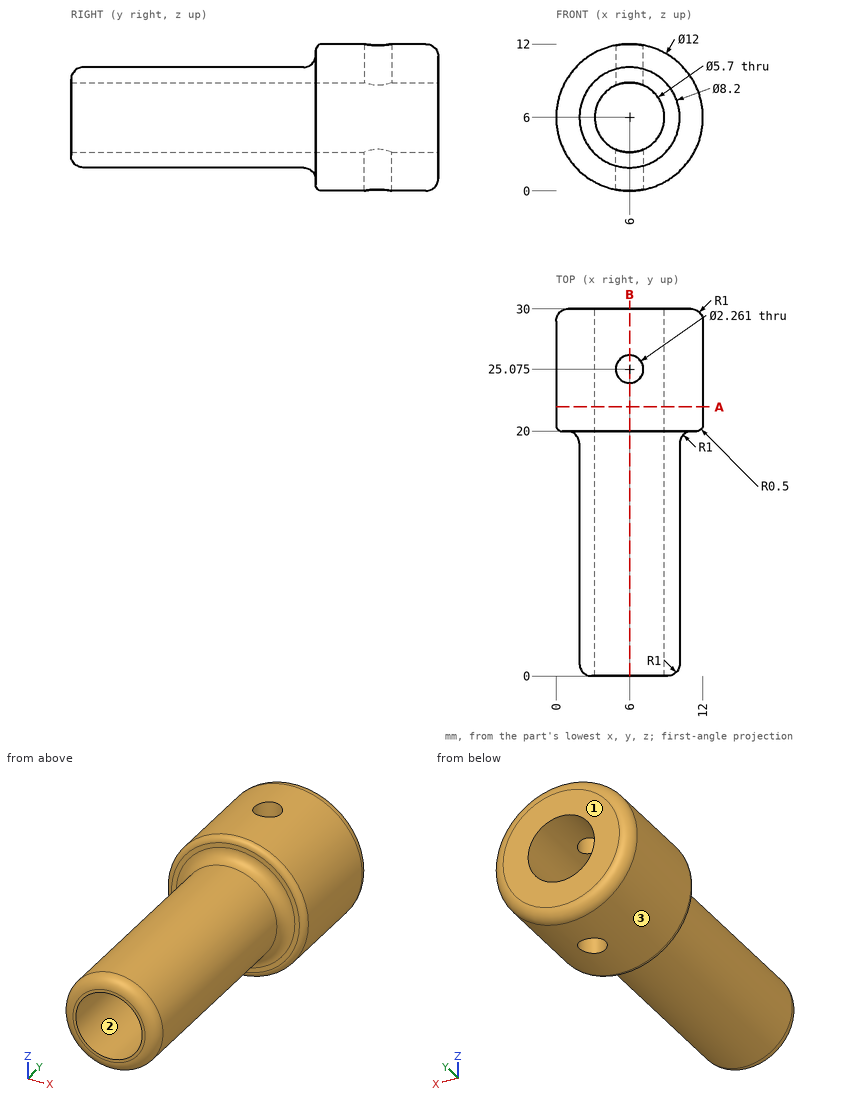
For this review, use the dimensioned drawing (mm, ordinates from the lowest corner) and the shaded views. Give positions to 0.01 mm unless a question says otherwise; leave off trailing zeros. Write each loop counter-clockwise with the first axis right and the second up, starting at its lowest first coordinate (ties: lowest second). Pieces come first, ordered by that corner, then holes. Notation, with made-up numbers: M 17.25,-27 L 30.25,-27 A15 cw 30.25,-17 Z; hole C 26,-29 d10. An arc over 180 degrees is marked long. Write item = value, one per line. Start each with the question number.
Q1. We need section B-B (x = 6). Give the number of separate pieces and of enclosed holes in the cut face.
Q2. Clearance check with flat-ended pins moving along their axes: pin 1 (1.5 mm diameter, centred on y = 14.5, z = 8.5, fed in from +X); pin 2 (1 mm diameter, centred on y = 15.5, z = 5, fed in from +X); pin 3 (5.5 mm diameter, centred on x = 4, z = 5.5, fed in from -Y); pin 4 (3 mm diameter, centred on x = 5.5, y = 4.5, fed in from +Z). State where each tip first meets the part, or that it passes through.
Q3. Mouldability with a two-part tool opening along Z and no side actions: class the marked faces 1, 2 and 3 as released by +Z, released by -Z, zero draft, split by the parting line, or undercut.
Q4. We need section A-A (y = 22). State the section outline as (x, z) points.
Q5. For line 1 (Z direction, x = 6, y = 9); line 2 (Y direction, x = 6, z = 1.6) (1 decimal); line 3 (Z direction, x = 7.25, y = 8.5) (1 decimal), list the stretches that pass through material, from the lowest coordinate up.
Result set:
q1.separate_pieces = 4
q1.enclosed_holes = 0
q2.pin_1 = 9.71
q2.pin_2 = 10.07
q2.pin_3 = 0
q2.pin_4 = 10.1
q3.face_1 = zero draft
q3.face_2 = undercut
q3.face_3 = split by the parting line
q4.outline = C 6,6 d12; hole C 6,6 d5.7
q5.line_1 = 1.9 to 3.15, 8.85 to 10.1
q5.line_2 = 19.7 to 23.9, 26.2 to 30
q5.line_3 = 2.1 to 3.4, 8.6 to 9.9
